Autodesk Inventor part; units mm, degrees
ref_plane "YZ Plane" through (0, 0, 0) normal (1, 0, 0) x (0, 1, 0)
ref_plane "XZ Plane" through (0, 0, 0) normal (0, 1, 0) x (-1, 0, 0)
ref_plane "XY Plane" through (0, 0, 0) normal (0, 0, 1) x (1, 0, 0)
sketch "Sketch1" plane through (0, 0, 0) normal (0, 0, 1) x (1, 0, 0)
  line L0 (-18.249, 5.8402) -> (8.251, 5.8402)
  line L1 (8.251, 5.8402) -> (8.251, -15.2598)
  line L2 (8.251, -15.2598) -> (-18.249, -15.2598)
  line L3 (-18.249, -15.2598) -> (-18.249, 5.8402)
  line L4 (-15.249, 2.8402) -> (5.251, 2.8402)
  line L5 (5.251, 2.8402) -> (5.251, -10.2598)
  line L6 (5.251, -10.2598) -> (-15.249, -10.2598)
  line L7 (-15.249, -10.2598) -> (-15.249, 2.8402)
  point P0 (0, 0)
  dimension "d0" = 20.5
  dimension "d1" = 13.1
  dimension "d2" = 3
  dimension "d3" = 3
  dimension "d4" = 5
  dimension "d5" = 3
extrude "Extrusion1" add sketch "Sketch1" along normal blind 2
sketch "Sketch2" plane through (-18.249, -15.2598, 0) normal (0, -1, 0) x (1, 0, 0)
  line L0 (-0.0474, 7) -> (26.5, 7)
  line L1 (26.5, 7) -> (26.5, -5)
  line L2 (26.5, -5) -> (-0.0474, -5)
  line L3 (-0.0474, -5) -> (-0.0474, 7)
  line L4 (0, 2) -> (26.5, 2)
  line L5 (26.5, 0) -> (0, 0)
  line L6 (26.5, 0) -> (26.5, 2)
  point P0 (18.249, 0)
  dimension "d8" = 5
  dimension "d9" = 5
  dimension "d10" = 0
extrude "Extrusion2" add sketch "Sketch2" along normal blind 1
fillet "Fillet1" radius 2 2 edges at (-4.999, -15.2598, 2) (-4.999, -15.2598, 0)
properties part number "switch mount test"
Read the model definition and answer for the solid it produces. Units are mm, in the model's axes. A direction names the side the tool comes from. Give positions to 0.01 mm unless a question says otherwise; leave off trailing zeros. Write each loop counter-clockwise with the first axis right and the second up, starting at its lowest first coordinate (ties: lowest second). Pieces come first, ordered by that corner, then holes. Notation, with made-up numbers: (-8, -3.5) - (38, -3.5) arc R19 ccw to (38, 26.5) - close; hole circle Ø2 at (-18.75, -40). An arc over 180 degrees is marked (long way). Use CSV: the item, a comma, the result in double quotes. Start each with the question number.
(1) Given P1, Ø3, axis at y = -8.5, z = 1.5, coming from the -X side; P2, Ø10, axis at x = -15, y = -5.5, coming from the -Z side; P3, Ø6, axis at y = -7.5, z = -2, coming from the +X side; P4, Ø5, axis at x = 4, z = -3.5, coming from the +Y side, each flat-ended and moving along its own axis, determine where each tip first touches the part or whether it passes through.
(2) For faces 1 (the flat face through (-5, -10.26, 1)), 2 (the flat face through (-5, -12, 2)), 3 (the flat face through (-5, -12, 0)), determine the directions among +Z, -Z, +X, -X, +Y, -Y from which every point of the face is accessible in a straight line to the end or side of a thin tool.
(3) Find section B-B (y = -0.75). Give the vertices of the cut face in (x, z), plus the area to 3 significant figures.
(4) Determine the mould class of faces 4 (the flat face through (-5, 2.84, 1)), 5 (the flat face through (-5, -15.26, 5)), 6 (the flat face through (5.251, -4, 1)), 7 (the flat face through (-18.249, -6, 1)) for opening direction X: +X half, -X half, draft (parallel to the pull), parting line (faces both ways), or undercut.
(5) Find section C-C (z = 0.75). Give the vertices of the cut face in (x, y), plus the area to 3 significant figures.
(6) Find section D-D (y = 3.75). Give the vertices of the cut face in (x, z).
(7) Consider line 1 along Y through (x, z) = (0.5, 0.75); line 2 along X through (y, z) = (-0.25, 1.25); line 3 along Z through (x, y) = (2, -12). Determine where each line is inside the solid, lowest interval first.
(8) Find section A-A (x = -11). Give the vertices of the cut face in (y, z).
Findings below:
1,P1,"x = -18.25"
1,P2,"z = 0"
1,P3,"x = 8.25"
1,P4,"y = -14.99"
2,face 1,"+Z, -Z"
2,face 2,"+Z, +X, -X, +Y"
2,face 3,"-Z, +X, -X, +Y"
3,outline,"(-18.25, 0) - (-15.25, 0) - (-15.25, 2) - (-18.25, 2) - close; (5.25, 0) - (8.25, 0) - (8.25, 2) - (5.25, 2) - close"
3,area,"12.0 mm2"
4,face 4,"undercut"
4,face 5,"draft"
4,face 6,"undercut"
4,face 7,"-X half"
5,outline,"(-18.3, -16.26) - (8.25, -16.26) - (8.25, 5.84) - (-18.25, 5.84) - (-18.25, -15.26) - (-18.3, -15.26) - close; hole (-15.25, -10.26) - (5.25, -10.26) - (5.25, 2.84) - (-15.25, 2.84) - close"
5,area,"317 mm2"
6,outline,"(-18.25, 0) - (8.25, 0) - (8.25, 2) - (-18.25, 2) - close"
7,line 1,"-16.26 to -10.26, 2.84 to 5.84"
7,line 2,"-18.25 to -15.25, 5.25 to 8.25"
7,line 3,"0 to 2"
8,outline,"(-16.26, -5) - (-15.26, -5) - (-15.26, -2) arc R2 cw to (-13.26, 0) - (-10.26, 0) - (-10.26, 2) - (-13.26, 2) arc R2 cw to (-15.26, 4) - (-15.26, 7) - (-16.26, 7) - close; (2.84, 0) - (5.84, 0) - (5.84, 2) - (2.84, 2) - close"
